Drawing for the job (mm, zero at the part's lowest x, y, z). A direction names the side the tool comes from. Give positions to 0.01 mm unless a question says otherwise; leave off trailing zeros. Order: outer loops, then holes, each group sorted by start corner. A loop starts at its lowest first (then second) coordinate and runs counter-clockwise, first axis right, second up. Notation, with made-up numbers: (-5, -40) - (33, -40) arc R23 ccw to (33, -12) - close; hole circle Ø7 at (78, 79). An arc over 180 degrees is marked (long way). One line per item, written item: value.
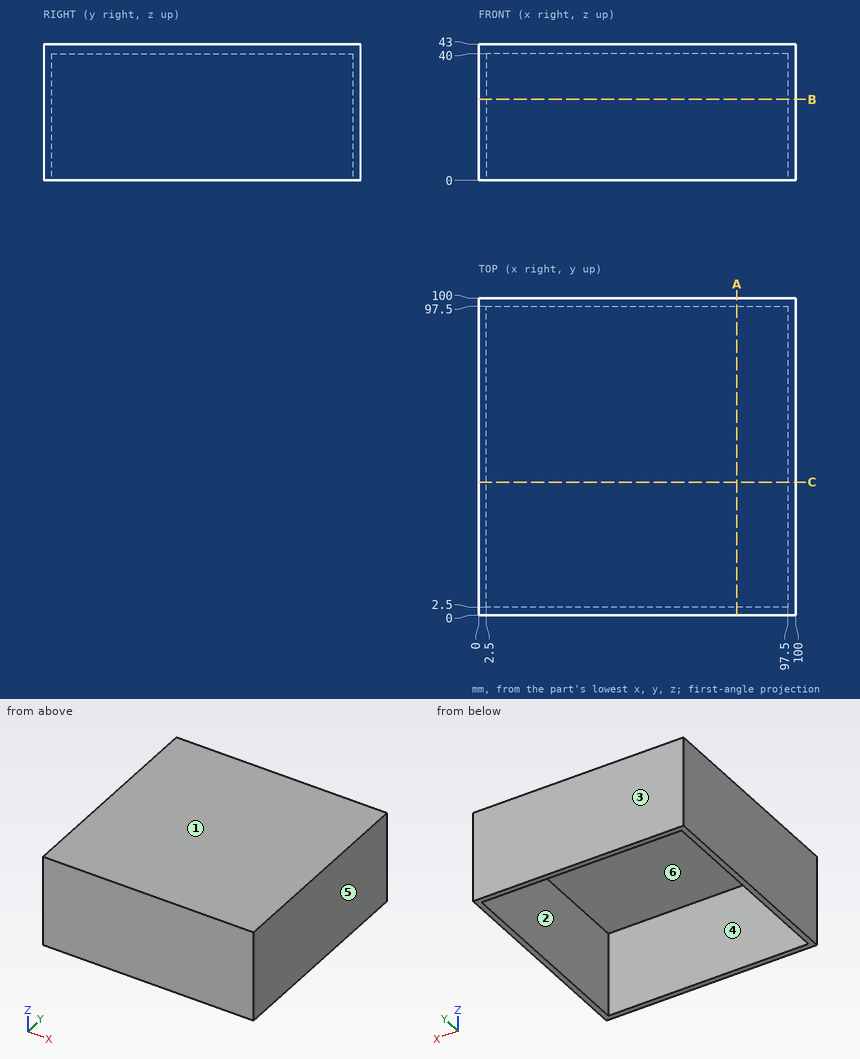
1) Cut at A-A, the plane x = 81.5. Give the cut face in (y, z), then the cut area to 3 significant figures.
Outcome:
outline: (0, 0) - (2.5, 0) - (2.5, 40) - (97.5, 40) - (97.5, 0) - (100, 0) - (100, 43) - (0, 43) - close
area: 500 mm^2
2) Which spindle directions (+Z, -Z, +X, -X, +Y, -Y) get a long thin tool onto all of the face, cutting with end or side? Do the marked faces 1 and 2. Say none if no direction does.
Outcome:
face 1: +Z, +X, -X, +Y, -Y
face 2: -Z
3) Cut at B-B, the plane z = 25.5. Give the cut face in (x, y).
Outcome:
outline: (0, 0) - (100, 0) - (100, 100) - (0, 100) - close; hole (2.5, 2.5) - (97.5, 2.5) - (97.5, 97.5) - (2.5, 97.5) - close
4) Mould opens along X. For the marked faces 3, 4, 5 and 6 say: released by +X, released by -X, zero draft, split by the parting line, or undercut.
Outcome:
face 3: zero draft
face 4: undercut
face 5: released by +X
face 6: undercut
5) Pin check, flat tips, straight feed: pin 1 (20 mm diameter, centred on y = 57.5, z = 27.5, fed in from -X); pin 2 (12 mm diameter, centred on x = 45, y = 31.5, fed in from -Z). Stop position of each tip, or through.
Outcome:
pin 1: stops at x = 0
pin 2: stops at z = 40
6) Drill centre lines: line 1 along X through (y, z) = (26, 23.5); line 2 along Z through (x, y) = (44.5, 9.5). Where is each one in solid material? Low to high. Write a range as from..to.
Outcome:
line 1: x = 0..2.5, 97.5..100
line 2: z = 40..43
